from build123d import *

# Parameters (mm, degrees)
F0_W     = 150
F0_H     = 50
F1_DEPTH = 5
F2_R     = 7.5
F3_DEPTH = 15
F4_R     = 4
F5_DEPTH = 150
F6_R     = 4
F7_DEPTH = 50


with BuildPart() as f1:
    # F0 (on Top) → F1 (new body)
    with BuildSketch(Plane.XY):
        with Locations((75, 25)):
            Rectangle(F0_W, F0_H)
    extrude(amount=F1_DEPTH)

    # F2 (on face) → F3 (join)
    with BuildSketch(Plane.XY.offset(5)):
        with Locations((45, 25)):
            Circle(F2_R)
        with Locations((75, 25)):
            Circle(F2_R)
        with Locations((105, 25)):
            Circle(F2_R)
    extrude(amount=F3_DEPTH)

    # F4 (on face) → F5 (join)
    with BuildSketch(Plane.XY.offset(20)):
        with Locations((45, 25)):
            Circle(F4_R)
        with Locations((105, 25)):
            Circle(F4_R)
    extrude(amount=F5_DEPTH)

    # F6 (on face) → F7 (join)
    with BuildSketch(Plane.XY.offset(20)):
        with Locations((75, 25)):
            Circle(F6_R)
    extrude(amount=F7_DEPTH)


solid = f1.part
Geometry check sheet. Reference: the model listing, model coordinates, mm. A direction names the side the tool comes from. Round coordinates to 2 decimals unless told otherwise and drop trailing zeros. Order: outer loops, then holes, each group sorted by start corner. A loop starts at its lowest first (then second) coordinate and runs counter-clockwise, first axis right, second up. Notation, with made-up numbers: M 49.25,82.25 L 56.25,82.25 A33 ccw 56.25,119.25 Z; hole C 83,41.5 d5. An arc over 180 degrees is marked long. Answer in a Markdown table with one row per item.
(1) Go/stop test with flat-tipped pins: P1, Ø1.5, axis at x = 130.5, y = 27.5, coming from the +Z side; P2, Ø3, axis at x = 45, z = 18.5, coming from the +Y side; P3, Ø8, axis at x = 113, y = 32.5, coming from the +Z side. Record where each tip stops, or that it passes through.
Responses:
| item | result |
|---|---|
| P1 | stops at z = 5 |
| P2 | stops at y = 32.5 |
| P3 | stops at z = 20 |
(2) Scan lines: probe 1 along X at (y, z) = (27, 32); probe 2 along Z at (x, y) = (71, 33.5); probe 3 along X at (y, z) = (21.5, 77). Record each from-to range of solid material in increasing order. Write a range as from..to.
Responses:
| item | result |
|---|---|
| probe 1 | x = 41.54..48.46, 71.54..78.46, 101.54..108.46 |
| probe 2 | z = 0..5 |
| probe 3 | x = 43.06..46.94, 103.06..106.94 |
(3) Sectioned sample at A-A, the plane y = 25. Record the cut outline in (x, z).
Responses:
| item | result |
|---|---|
| outline | M 0,0 L 150,0 L 150,5 L 112.5,5 L 112.5,20 L 109,20 L 109,170 L 101,170 L 101,20 L 97.5,20 L 97.5,5 L 82.5,5 L 82.5,20 L 79,20 L 79,70 L 71,70 L 71,20 L 67.5,20 L 67.5,5 L 52.5,5 L 52.5,20 L 49,20 L 49,170 L 41,170 L 41,20 L 37.5,20 L 37.5,5 L 0,5 Z |
(4) Tool access check on faces 1 (the face through (150, 25, 2)), 2 (the face through (104.024, 32.436, 12.395)), 3 (the face through (75, 25, 70)). Record the directions out of +Z, -Z, +X, -X, +Y, -Y that give a thin tool (end or side, any length) a straight path to the whole face; none if there is none.
Responses:
| item | result |
|---|---|
| face 1 | +Z, -Z, +X, +Y, -Y |
| face 2 | +Z |
| face 3 | +Z, +Y, -Y |
(5) Draft check along X on faces 4 (the face through (45, 25, 170)), 5 (the face through (0, 25, 2)), 6 (the face through (48, 22, 20)). Enter one of: released by +X, released by -X, zero draft, split by the parting line, or undercut.
Responses:
| item | result |
|---|---|
| face 4 | zero draft |
| face 5 | released by -X |
| face 6 | undercut |
(6) Sectioned sample at C-C, the plane z = 143. Record the cut outline in (x, y).
Responses:
| item | result |
|---|---|
| outline | C 45,25 d8; C 105,25 d8 |
(7) Sectioned sample at B-B, the plane x = 45. Record the cut outline in (y, z).
Responses:
| item | result |
|---|---|
| outline | M 0,0 L 50,0 L 50,5 L 32.5,5 L 32.5,20 L 29,20 L 29,170 L 21,170 L 21,20 L 17.5,20 L 17.5,5 L 0,5 Z |
(8) Sectioned sample at D-D, the plane x = 75. Record the cut outline in (y, z).
Responses:
| item | result |
|---|---|
| outline | M 0,0 L 50,0 L 50,5 L 32.5,5 L 32.5,20 L 29,20 L 29,70 L 21,70 L 21,20 L 17.5,20 L 17.5,5 L 0,5 Z |
